Check sheet for the modelled part. Datum: model origin and axes. Units: mm. A direction names the side the tool comes from. Coordinates: 2 decimals unless noted, no trailing zeros. Write each loop counter-clockwise with the first axis right and the second up, starting at its lowest first coordinate (ties: lowest second). Pieces come first, ordered by that corner, then holes. Notation, with made-up numbers: (-1, 26.5) - (28, 26.5) arc R11 cw to (28, 31.5) - close; hole circle Ø9 at (-6.75, 27). An arc over 180 degrees is marked (long way). Answer as CSV lines item,"result". Start each with the question number.
from build123d import *

# Parameters (mm, degrees)
SKETCH2_R                              = 11.176
BOSS_EXTRUDE1_DEPTH                    = 9.144
SKETCH3_R                              = 8.89
SKETCH3_R_2                            = 3.1115
CUT_EXTRUDE1_DEPTH                     = 0.635
CHAMFER1_SIZE                          = 0.254
CHAMFER2_SIZE                          = 1.27
BOSS_EXTRUDE2_START                    = 1.27
SKETCH10_R                             = 3.1115
SKETCH10_R_2                           = 1.5875
BOSS_EXTRUDE2_DEPTH                    = 1.27
CHAMFER3_SIZE                          = 0.254
F_2_56_TAPPED_HOLE3_D                  = 1.778
F_2_56_TAPPED_HOLE3_DEPTH              = 11.43
F_2_56_TAPPED_HOLE3_CSINK_D            = 2.54
F_2_56_TAPPED_HOLE3_CSINK_ANGLE        = 90
F_2_56_TAPPED_HOLE3_TIP                = 0.53416509
F_29_0_136_DIAMETER_HOLE1_D            = 3.4544
B_0_238_DIAMETER_HOLE1_D               = 6.0452
B_0_238_DIAMETER_HOLE1_DEPTH           = 4.445
B_0_238_DIAMETER_HOLE1_TIP             = 1.816161307
F_1_16_0_0625_DIAMETER_HOLE1_OUTLINE_R = 0.79375
F_1_16_0_0625_DIAMETER_HOLE1_DEPTH     = 3.359771909


# Read off the part's stored shape, not the designer's step: 1/16 (0.0625) Diameter Hole1
with BuildPart() as part:
    # Sketch2 → Boss-Extrude1 (new body)
    with BuildSketch(Plane(origin=(0, 0, 0), x_dir=(1, 0, 0), z_dir=(0, 1, 0))):
        with Locations(Location((0, 0, 0), (0, 0, 270))):
            Circle(SKETCH2_R)
    extrude(amount=BOSS_EXTRUDE1_DEPTH)

    # Sketch3 → Cut-Extrude1 (cut)
    with BuildSketch(Plane(origin=(0, 9.144, 0), x_dir=(1, 0, 0), z_dir=(0, 1, 0))):
        with Locations(Location((0, 0, 0), (0, 0, 270))):
            Circle(SKETCH3_R)
        with Locations(Location((0, 0, 0), (0, 0, 270))):
            Circle(SKETCH3_R_2, mode=Mode.SUBTRACT)
    extrude(amount=-CUT_EXTRUDE1_DEPTH, mode=Mode.SUBTRACT)

    # Chamfer1
    chamfer1_edges = [part.edges().sort_by_distance(p)[0] for p in [
        (0, 9.144, -11.176),
    ]]
    chamfer(chamfer1_edges, length=CHAMFER1_SIZE)

    # Chamfer2
    chamfer2_edges = [part.edges().sort_by_distance(p)[0] for p in [
        (0, 0, -11.176),
    ]]
    chamfer(chamfer2_edges, length=CHAMFER2_SIZE)

    # Sketch10 → Boss-Extrude2 (add)
    with BuildSketch(Plane(origin=(0, 9.144, 0), x_dir=(1, 0, 0), z_dir=(0, 1, 0)).offset(BOSS_EXTRUDE2_START)):
        with Locations(Location((0, 0, 0), (0, 0, 270))):
            Circle(SKETCH10_R)
        with Locations(Location((0, 0, 0), (0, 0, 270))):
            Circle(SKETCH10_R_2, mode=Mode.SUBTRACT)
    extrude(amount=-BOSS_EXTRUDE2_DEPTH)

    # Chamfer3
    chamfer3_edges = [part.edges().sort_by_distance(p)[0] for p in [
        (0, 10.414, -3.1115),
    ]]
    chamfer(chamfer3_edges, length=CHAMFER3_SIZE)

    # #2-56 Tapped Hole3
    with Locations(Plane(origin=(-8.082230509, 0, 8.082230509), x_dir=(0, -1, 0), z_dir=(-0.7071067811865488, 0, 0.7071067811865464))):
        with Locations((-3.175, 0)):
            CounterSinkHole(F_2_56_TAPPED_HOLE3_D / 2, F_2_56_TAPPED_HOLE3_CSINK_D / 2, depth=F_2_56_TAPPED_HOLE3_DEPTH, counter_sink_angle=F_2_56_TAPPED_HOLE3_CSINK_ANGLE)
            with Locations((0, 0, -(F_2_56_TAPPED_HOLE3_DEPTH + F_2_56_TAPPED_HOLE3_TIP / 2))):  # 118° drill point
                Cone(0, F_2_56_TAPPED_HOLE3_D / 2, F_2_56_TAPPED_HOLE3_TIP, mode=Mode.SUBTRACT)

    # #29 (0.136) Diameter Hole1 (through all)
    with Locations(Plane(origin=(0, 0, 0), x_dir=(-1, 0, 0), z_dir=(0, -1, 0))):
        with Locations((0, 0)):
            Hole(F_29_0_136_DIAMETER_HOLE1_D / 2)

    # B (0.238) Diameter Hole1
    with Locations(Plane(origin=(0, 9.144, 0), x_dir=(1, 0, 0), z_dir=(0, 1, 0))):
        with Locations((-6.985, 0), (0, 6.985), (0, -6.985), (6.985, 0)):
            Hole(B_0_238_DIAMETER_HOLE1_D / 2, depth=B_0_238_DIAMETER_HOLE1_DEPTH)
            with Locations((0, 0, -(B_0_238_DIAMETER_HOLE1_DEPTH + B_0_238_DIAMETER_HOLE1_TIP / 2))):  # 118° drill point
                Cone(0, B_0_238_DIAMETER_HOLE1_D / 2, B_0_238_DIAMETER_HOLE1_TIP, mode=Mode.SUBTRACT)

    # 1/16 (0.0625) Diameter Hole1 outline → 1/16 (0.0625) Diameter Hole1 (cut)
    with BuildSketch(Plane(origin=(0, 0, 0), x_dir=(1, 0, 0), z_dir=(0, 1, 0))):
        with Locations((-6.985, 0)):
            Circle(F_1_16_0_0625_DIAMETER_HOLE1_OUTLINE_R)
        with Locations((0, -6.985)):
            Circle(F_1_16_0_0625_DIAMETER_HOLE1_OUTLINE_R)
        with Locations((6.985, 0)):
            Circle(F_1_16_0_0625_DIAMETER_HOLE1_OUTLINE_R)
        with Locations((0, 6.985)):
            Circle(F_1_16_0_0625_DIAMETER_HOLE1_OUTLINE_R)
    extrude(amount=F_1_16_0_0625_DIAMETER_HOLE1_DEPTH, mode=Mode.SUBTRACT)


solid = part.part
(1) Go/stop test with flat-tipped pins: P1, Ø5.5, axis at x = -6.985, z = 0, coming from the +Y side; P2, Ø1.5, axis at x = -4, z = 1, coming from the +Y side; P3, Ø3, axis at x = -3, y = 2.5, coming from the +Z side. Record where each tip stops, or that it passes through.
(2) Cross-section at C-C on y = 7.75. Record the boundary of the cut face in (x, z) (3 decimals).
(3) Release check for a two-part mould opening along Y. For faces 1 (the face through (-2, 10.414, 0)), 2 (the face through (-4.94, 3.585, 3.825)), 3 (the face through (0.655, 6.89, 9.936)) record: pulls with the +Y half, pulls with the -Y half, needs draft (parallel to the pull), parting line crosses it, or undercut.
(4) Tool access check on faces 4 (the face through (6.33, 8.83, -6.24)), 5 (the face through (-7.6, 1.7, 0.5)). Record the directions out of +Z, -Z, +X, -X, +Y, -Y that give a thin tool (end or side, any length) a straight path to the whole face; none if there is none.
(5) Cross-section at A-A on z = 0. State how many separate pieces and enclosed holes the cut face has, plus the area to 3 significant figures.
(6) Material ranges on probe 1 along X at (y, z) = (8, -2.5); probe 2 along Z at (x, y) = (1, 3); probe 3 along Y at (x, z) = (3.75, 5), recorded low to high. Write a range as from..to.
Checked values:
1,P1,"y = 4.54"
1,P2,"y = 8.51"
1,P3,"z = 11.07"
2,outline,"circle Ø22.352 at (0, 0); hole circle Ø6.045 at (-6.985, 0); hole circle Ø6.045 at (0, -6.985); hole circle Ø6.045 at (0, 6.985); hole circle Ø3.454 at (0, 0); hole circle Ø6.045 at (6.985, 0)"
3,face 1,"pulls with the +Y half"
3,face 2,"undercut"
3,face 3,"needs draft"
4,face 4,"+Y"
4,face 5,"+Y, -Y"
5,separate pieces,"4"
5,enclosed holes,"0"
5,area,"98.9 mm^2"
6,probe 1,"-10.89..-8.68, -5.29..5.29, 8.68..10.89"
6,probe 2,"-11.13..-1.41, 1.41..11.13"
6,probe 3,"0..8.51"
